Input: part model. Units: mm. Frame: model coordinates. Face numbers are marked on the shaded views. Round coordinates to 2 decimals unless told otherwise and drop trailing zeros. Loops run counter-clockwise (first coordinate to the right, second up) from the corner with the lowest first, then second, coordinate; pieces in that order, holes last. Notation, with made-up numbers: (51.5, 42.25) -> (82.5, 42.25) arc R30 cw to (82.5, 68.25) -> close; hole circle Ø6 at (-1.5, -5). An arc over 180 degrees is marked (long way). Answer as a JSON object with one key per item and string values.
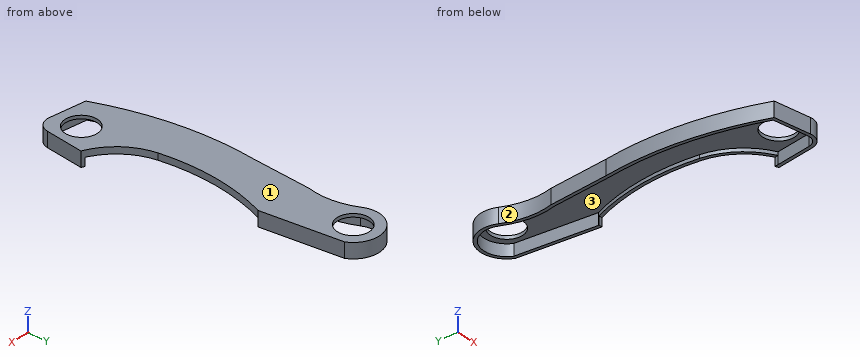
```python
from build123d import *

# Parameters (mm, degrees)
BOSS_EXTRUDE1_DEPTH     = 3.429
FILLET1_R               = 3.175
SKETCH2_R               = 2.921
CUT_EXTRUDE1_DEPTH      = 110.435380853
SHELL2_OUTLINE_R        = 3.683
SHELL2_DEPTH            = 2.667
CUT_EXTRUDE2_REACH      = 111.435
SKETCH3_R               = 3.683
CUT_EXTRUDE3_REACH      = 80.749
SKETCH4_W               = 1.905
SKETCH4_H               = 36.940823868
CUT_EXTRUDE4_DEPTH      = 110.435380853
CUT_EXTRUDE4_DEPTH_BACK = 1.778
CUT_EXTRUDE5_DEPTH      = 0.127


# Read off the part's stored shape, not the designer's step: Shell2
with BuildPart() as part:
    # Sketch1 → Boss-Extrude1 (new body)
    with BuildSketch(Plane.XY):
        with BuildLine():
            Line((62.7345016, 80.577747087), (64.726975666, 62.289747087))
            ThreePointArc((64.726975666, 62.289747087), (61.454694837, 49.585208184), (61.721936912, 36.468740968))
            ThreePointArc((61.721936912, 36.468740968), (64.516939118, 30.014666788), (70.081936923, 25.713747087))
            Line((70.081936923, 25.713747087), (68.536975666, 13.775747087))
            Line((68.536975666, 13.775747087), (56.940284848, 15.553747087))
            ThreePointArc((56.940284848, 15.553747087), (52.413143628, 32.787644792), (52.280975666, 50.605747087))
            Line((52.280975666, 50.605747087), (53.296975666, 64.302418224))
            ThreePointArc((53.296975666, 64.302418224), (53.653310061, 69.952097941), (52.044858214, 75.37968836))
            ThreePointArc((52.044858214, 75.37968836), (54.7617878, 83.382894736), (62.7345016, 80.577747087))
        make_face()
    extrude(amount=BOSS_EXTRUDE1_DEPTH)

    # Fillet1
    fillet1_edges = [part.edges().sort_by_distance(p)[0] for p in [
        (68.536975666, 13.775747087, 1.7145),
    ]]
    fillet(fillet1_edges, radius=FILLET1_R)

    # Sketch2 → Cut-Extrude1 (cut, through all)
    with BuildSketch(Plane.XY.offset(3.429)):
        with Locations((57.360975666, 78.037747087)):
            Circle(SKETCH2_R)
        with Locations((63.826413409, 20.421081821)):
            Circle(SKETCH2_R)
    extrude(amount=-CUT_EXTRUDE1_DEPTH, mode=Mode.SUBTRACT)

    # Shell2 outline → Shell2 (cut)
    with BuildSketch(Plane.XY):
        with BuildLine():
            ThreePointArc((61.991345759, 80.363397827), (55.039508366, 82.670215989), (52.726411733, 75.72046512))
            ThreePointArc((52.726411733, 75.72046512), (54.406890906, 70.069245661), (54.052294982, 64.184132803))
            Line((54.052294982, 64.184132803), (53.039664753, 50.532889471))
            ThreePointArc((53.039664753, 50.532889471), (53.139176681, 33.111364087), (57.487066991, 16.240818773))
            Line((57.487066991, 16.240818773), (65.439706148, 15.021523317))
            ThreePointArc((65.439706148, 15.021523317), (67.256047768, 15.478396864), (68.198436672, 17.096955938))
            Line((68.198436672, 17.096955938), (69.253887741, 25.252483979))
            ThreePointArc((69.253887741, 25.252483979), (63.739946861, 29.77722029), (60.969261533, 36.349897487))
            ThreePointArc((60.969261533, 36.349897487), (60.686685648, 49.576935849), (63.948610548, 62.398567528))
            Line((63.948610548, 62.398567528), (61.991345759, 80.363397827))
        make_face()
        with Locations((63.826413409, 20.421081821)):
            Circle(SHELL2_OUTLINE_R, mode=Mode.SUBTRACT)
        with Locations((57.360975666, 78.037747087)):
            Circle(SHELL2_OUTLINE_R, mode=Mode.SUBTRACT)
    extrude(amount=SHELL2_DEPTH, mode=Mode.SUBTRACT)

    # Sketch3 → Cut-Extrude2 (cut, up to next)
    with BuildSketch(Plane(origin=(0, 0, 0), x_dir=(-1, 0, 0), z_dir=(0, 0, -1)), mode=Mode.PRIVATE) as cut_extrude2_sk1:
        with Locations((-57.360975666, 78.037747087)):
            Circle(SKETCH3_R)
    cut_extrude2_tool1 = extrude(cut_extrude2_sk1.sketch, amount=-CUT_EXTRUDE2_REACH, mode=Mode.PRIVATE) & part.part
    # Sketch3 → Cut-Extrude2 (cut, up to next)
    with BuildSketch(Plane(origin=(0, 0, 0), x_dir=(-1, 0, 0), z_dir=(0, 0, -1)), mode=Mode.PRIVATE) as cut_extrude2_sk2:
        with Locations((-63.826413409, 20.421081821)):
            Circle(SKETCH3_R)
    cut_extrude2_tool2 = extrude(cut_extrude2_sk2.sketch, amount=-CUT_EXTRUDE2_REACH, mode=Mode.PRIVATE) & part.part
    add(cut_extrude2_tool1.solids().sort_by_distance((57.360976, 78.037747, 0))[0], mode=Mode.SUBTRACT)
    add(cut_extrude2_tool2.solids().sort_by_distance((63.826413, 20.421082, 0))[0], mode=Mode.SUBTRACT)

    # Sketch4 → Cut-Extrude3 (cut, up to next)
    with BuildSketch(Plane(origin=(70.674520745, 7.699975379, 0), x_dir=(0, 0, -1), z_dir=(0.9941172894005426, 0.10830888659255154, 0)), mode=Mode.PRIVATE) as cut_extrude3_sk1:
        with Locations((-0.9525, 36.44239593)):
            Rectangle(SKETCH4_W, SKETCH4_H)
    cut_extrude3_tool1 = extrude(cut_extrude3_sk1.sketch, amount=-CUT_EXTRUDE3_REACH, mode=Mode.PRIVATE) & part.part
    add(cut_extrude3_tool1.solids().sort_by_distance((66.727485, 43.927991, 0.9525))[0], mode=Mode.SUBTRACT)

    # Sketch5 → Cut-Extrude4 (cut, two sides: drawn at the far end of the back side and taken through both)
    with BuildSketch(Plane(origin=(0, 0, 0), x_dir=(-1, 0, 0), z_dir=(0, 0, -1)).offset(-CUT_EXTRUDE4_DEPTH_BACK)):
        with BuildLine():
            Line((-69.357085228, 26.049896593), (-69.253887741, 25.252483979))
            ThreePointArc((-69.253887741, 25.252483979), (-68.949955482, 25.401641313), (-68.649499804, 25.557683339))
            Line((-68.649499804, 25.557683339), (-68.727995169, 25.566235394))
            Line((-68.727995169, 25.566235394), (-68.633052886, 26.437666796))
            ThreePointArc((-68.633052886, 26.437666796), (-68.992244892, 26.238508503), (-69.357085228, 26.049896593))
        make_face()
    extrude(amount=CUT_EXTRUDE4_DEPTH + CUT_EXTRUDE4_DEPTH_BACK, mode=Mode.SUBTRACT)

    # Sketch6 → Cut-Extrude5 (cut)
    with BuildSketch(Plane(origin=(0, 0, 1.778), x_dir=(-1, 0, 0), z_dir=(0, 0, -1))):
        with BuildLine():
            Line((-69.357085228, 26.049896593), (-69.253887741, 25.252483979))
            ThreePointArc((-69.253887741, 25.252483979), (-68.949955482, 25.401641313), (-68.649499804, 25.557683339))
            Line((-68.649499804, 25.557683339), (-68.727995169, 25.566235394))
            Line((-68.727995169, 25.566235394), (-68.633052886, 26.437666796))
            ThreePointArc((-68.633052886, 26.437666796), (-68.992244892, 26.238508503), (-69.357085228, 26.049896593))
        make_face()
    extrude(amount=-CUT_EXTRUDE5_DEPTH, mode=Mode.SUBTRACT)


solid = part.part
```
1) Section B-B, the plane y = 44.5. Output: boundary loops of the cut face in (x, z) (3 decimals).
Output:
{"outline": "(51.825, 0) -> (52.587, 0) -> (52.587, 2.667) -> (60.371, 2.667) -> (60.371, 1.905) -> (61.133, 1.905) -> (61.133, 3.429) -> (51.825, 3.429) -> close"}
2) Draft query along Y for the marked faces 1, 2 and 3. Return one class per face: +Y half, -Y half, draft (parallel to the pull), parting line (faces both ways), or undercut.
Output:
{"face 1": "draft", "face 2": "undercut", "face 3": "undercut"}
3) Section A-A, the plane x = 56. Output: boundary loops of the cut face in (y, z), plus the area to 3 significant figures.
Output:
{"outline": "(18.03, 0) -> (20.39, 0) -> (20.39, 2.67) -> (74.62, 2.67) -> (74.62, 3.43) -> (18.03, 3.43) -> close; (81.46, 2.67) -> (83.04, 2.67) -> (83.04, 0) -> (83.82, 0) -> (83.82, 3.43) -> (81.46, 3.43) -> close", "area": "53.3 mm^2"}
4) Contact query for flat-ended pins moving along their axis: P1, Ø2, axis at y = 52, z = 2, coming from the +X side; P2, Ø5, axis at x = 60, y = 62.5, coming from the -Z side. Output: stop coordinate, or through.
Output:
{"P1": "stops at x = 61.98", "P2": "stops at z = 2.67"}
5) Section C-C, the plane y = 69.5. Output: boundary loops of the cut face in (x, z).
Output:
{"outline": "(53.7, 0) -> (54.46, 0) -> (54.46, 2.67) -> (63.17, 2.67) -> (63.17, 0) -> (63.94, 0) -> (63.94, 3.43) -> (53.7, 3.43) -> close"}
6) Ray query, probe 1 along Z at (x, y) = (57, 37); probe 2 along Y at (x, z) = (60.25, 1.4); probe 3 along Y at (x, z) = (60.75, 0.2). Return the intervals inside material, ascending.
Output:
{"probe 1": "z = 2.67 to 3.43", "probe 2": "y = 15.05 to 15.82, 82.34 to 83.23", "probe 3": "y = 14.97 to 15.74, 81.96 to 82.92"}
